Autodesk Inventor part; units mm, degrees
ref_plane "YZ Plane" through (0, 0, 0) normal (1, 0, 0) x (0, 1, 0)
ref_plane "XZ Plane" through (0, 0, 0) normal (0, 1, 0) x (-1, 0, 0)
ref_plane "XY Plane" through (0, 0, 0) normal (0, 0, 1) x (1, 0, 0)
sketch "Sketch1" plane through (0, 0, 0) normal (0, 1, 0) x (-1, 0, 0)
  line L0 (0, 0) -> (0, -34.15) construction
  arc A0 (6.6649, -3.975) -> (-7.575, -7.575) centre (0, -7.575) ccw construction
  arc A1 (-7.575, -26.575) -> (6.6649, -30.175) centre (0, -26.575) ccw construction
  line L1 (4.075, -7.575) -> (4.075, -26.575) construction
  arc A2 (-4.075, -26.575) -> (4.075, -26.575) centre (0, -26.575) ccw construction
  line L2 (-4.075, -26.575) -> (-4.075, -7.575) construction
  arc A3 (4.075, -7.575) -> (-4.075, -7.575) centre (0, -7.575) ccw construction
  line L3 (9.1649, -3.975) -> (9.1649, -30.175) construction
  line L4 (9.1649, -3.975) -> (6.6649, -3.975) construction
  line L5 (9.1649, -30.175) -> (6.6649, -30.175) construction
  line L6 (-10.575, -14.075) -> (-10.575, -20.075) construction
  line L7 (0, -17.075) -> (-19.3792, -17.075) construction
  line L8 (-4.075, -20.075) -> (-4.075, -24.075) construction
  line L9 (-10.575, -20.075) -> (-7.575, -21.8932) construction
  line L10 (-10.575, -14.075) -> (-7.575, -12.2568) construction
  line L11 (-7.575, -7.575) -> (-7.575, -12.2568) construction
  line L12 (-7.575, -21.8932) -> (-7.575, -26.575) construction
  line L13 (-10.575, -17.075) -> (-16.875, -17.075) construction
  line L14 (-10.575, -14.075) -> (-14.875, -14.075) construction
  line L15 (-16.875, -16.075) -> (-16.875, -18.075) construction
  line L16 (-14.875, -20.075) -> (-10.575, -20.075) construction
  arc A4 (-14.875, -14.075) -> (-16.875, -16.075) centre (-14.875, -16.075) ccw construction
  arc A5 (-16.875, -18.075) -> (-14.875, -20.075) centre (-14.875, -18.075) ccw construction
  line L17 (-6.7059, -17.075) -> (-6.7059, -23.075) construction
  line L18 (-6.7059, -17.075) -> (-6.7059, -11.075) construction
  line L19 (-7.575, -11.075) -> (-14.875, -11.075) construction
  line L20 (-16.875, -13.075) -> (-16.875, -21.075) construction
  line L21 (-14.875, -23.075) -> (-7.575, -23.075) construction
  arc A6 (-14.875, -11.075) -> (-16.875, -13.075) centre (-14.875, -13.075) ccw construction
  arc A7 (-16.875, -21.075) -> (-14.875, -23.075) centre (-14.875, -21.075) ccw construction
  line L22 (19.3047, -16.075) -> (19.3047, -18.075) construction
  line L23 (17.3047, -14.075) -> (13.3047, -14.075) construction
  line L24 (17.3047, -20.075) -> (13.3047, -20.075) construction
  line L25 (9.1649, -16.075) -> (9.1649, -22.575) construction
  line L26 (9.1649, -17.075) -> (9.1649, -11.575) construction
  line L27 (9.1649, -11.575) -> (13.3047, -14.075) construction
  line L28 (9.1649, -22.575) -> (13.3047, -20.075) construction
  arc A8 (19.3047, -16.075) -> (17.3047, -14.075) centre (17.3047, -16.075) ccw construction
  arc A9 (17.3047, -20.075) -> (19.3047, -18.075) centre (17.3047, -18.075) ccw construction
  line L29 (9.1649, -30.175) -> (9.1649, -26.175) construction
  line L30 (9.1649, -3.975) -> (9.1649, -7.975) construction
  line L31 (9.1649, -24.9114) -> (13.8618, -22.075) construction
  line L32 (13.8618, -22.075) -> (17.3047, -22.075) construction
  arc A10 (17.3047, -22.075) -> (21.3047, -18.075) centre (17.3047, -18.075) ccw construction
  line L33 (21.3047, -18.075) -> (21.3047, -16.075) construction
  arc A11 (21.3047, -16.075) -> (17.3047, -12.075) centre (17.3047, -16.075) ccw construction
  line L34 (17.3047, -12.075) -> (13.8618, -12.075) construction
  line L35 (13.8618, -12.075) -> (9.1649, -9.2386) construction
  point P0 (7.575, -17.075)
  point P1 (-4.075, -10.075)
  point P2 (19.3047, -14.075)
  point P3 (19.3047, -20.075)
  dimension "d0" = 34.15
  dimension "d1" = 15.15
  dimension "d5" = 6
  dimension "d7" = 4
  dimension "d8" = 2.5
  dimension "d9" = 3.5
  dimension "d10" = 8.15
  dimension "d12" = 2
  dimension "d14" = 6
  dimension "d15" = 6
  dimension "d16" = 2
  dimension "d18" = 6
  dimension "d19" = 6
  dimension "d20" = 5.5
  dimension "d21" = 5.5
  dimension "d23" = 4
  dimension "d24" = 4
  dimension "d25" = 2
sketch "Sketch3" plane through (0, 0, 0) normal (0, 1, 0) x (-1, 0, 0)
  arc A0 (6.6649, -3.975) -> (-7.575, -7.575) centre (0, -7.575) ccw construction
  arc A1 (-7.575, -26.575) -> (6.6649, -30.175) centre (0, -26.575) ccw construction
  arc A2 (-4.075, -26.575) -> (4.075, -26.575) centre (0, -26.575) ccw
  line L0 (4.075, -7.575) -> (4.075, -26.575)
  arc A3 (4.075, -7.575) -> (-4.075, -7.575) centre (0, -7.575) ccw
  line L1 (-4.075, -26.575) -> (-4.075, -7.575)
  line L2 (9.1649, -3.975) -> (9.1649, -30.175) construction
  line L3 (-10.575, -14.075) -> (-10.575, -20.075) construction
  line L4 (-16.875, -16.075) -> (-16.875, -18.075) construction
  arc A4 (8.836, -1.765) -> (-4.3309, 2.0725) centre (0, -7.575) ccw
  arc A5 (-4.3309, -36.2225) -> (8.836, -32.385) centre (0, -26.575) ccw
  line L5 (9.1649, -2.8638) -> (9.1649, -31.2862)
  arc A6 (9.1649, -2.8638) -> (8.836, -1.765) centre (7.1649, -2.8638) ccw
  arc A7 (8.836, -32.385) -> (9.1649, -31.2862) centre (7.1649, -31.2862) ccw
  line L6 (-12.075, -10.8843) -> (-12.075, -24.6972)
  ellipse E0 centre (0, -17.075) end of major axis (0, -37.15) minor radius 14.4147 (-4.3309, 2.0725) -> (-4.3309, -36.2225) ccw
  point P0 (0, 0)
  point P1 (9.1649, -2.2991)
  point P2 (9.1649, -31.8509)
  dimension "d26" = 3
  dimension "d27" = 3
  dimension "d28" = 2
  dimension "d29" = 6.5
  dimension "d30" = 8
extrude "Extrusion1" add sketch "Sketch3" along normal blind 1
ref_plane "Work Plane1" through (0, 1, 3) normal (1, 0, 0) x (0, 0, -1)
sketch "Sketch7" plane through (0, 1, 3) normal (1, 0, 0) x (0, 0, -1)
  line L0 (40.15, 0) -> (40.15, -1)
  line L1 (40.15, -1) -> (33.65, -1)
  line L2 (33.65, -1) -> (33.65, 0)
  line L3 (33.65, 0) -> (40.15, 0)
  line L4 (0, -1) -> (0, 0)
  line L5 (0, 0) -> (6.5, 0)
  line L6 (6.5, 0) -> (6.5, -1)
  line L7 (6.5, -1) -> (0, -1)
  line L8 (40.15, -1) -> (35.385, -1) construction
  line L9 (40.15, -1) -> (40.15, -0.5) construction
  line L10 (40.15, -1) -> (40.15, 0) construction
  line L11 (4.765, 0) -> (0, 0) construction
  line L12 (40.15, -0.5) -> (0, 0)
  line L13 (0, 0) -> (40.15, 0)
  line L14 (40.15, 0) -> (40.15, -0.5)
  point P0 (3, -1)
  point P1 (39.2225, -1)
  point P2 (0.9275, 0)
extrude "Extrusion2" cut sketch "Sketch7" along normal blind 20 and the other way blind 20 contours L0 L12 L2 L3 | L2 L12 L6 L13 | L6 L12 L5
properties part number "SPD_MTB_cleat_new_1mm_05mm"
Here's how the part is built. I have some questions about the finished solid (model axes, mm). A direction names the side the tool comes from. Coordinates: 2 decimals unless noted, no trailing zeros. Order: outer loops, then holes, each group sorted by start corner. A loop starts at its lowest first (then second) coordinate and runs counter-clockwise, first axis right, second up.
Item 1: I need wall thicknesses on probe 1 along Z at (x, y) = (0, 0.45); probe 2 along X at (y, z) = (0.85, -5.5); probe 3 along X at (y, z) = (0.25, -19) (3 decimals). Which ranges of each line are inside material? Lowest first, please.
Response values:
probe 1: z = -37.15 to -30.65, -3.5 to 3
probe 2: x = -9.16 to -3.51, 3.51 to 11.78
probe 3: x = -9.165 to -4.075, 4.075 to 14.348
Item 2: Which directions (+Z, -Z, +X, -X, +Y, -Y) give clear straight access to the entire face, cutting with the end or side of a thin tool? Please do faces 5 (the face through (-9.165, 0.4, -16.9)), 6 (the face through (-4.075, 0.3, -16.9)).
Response values:
face 5: +Z, -Z, -X, +Y, -Y
face 6: +Y, -Y
Item 3: Thinking about a two-plate mould opening in X: for faces 1 (the face through (-9.079, 0.464, -2.283)), 2 (the face through (-2.859, 0.493, 2.606)), 3 (the face through (4.075, 0.3, -17.2)), 4 (the face through (5, 0, -17)), which applies, pulls with the +X half, pulls with the -X half, needs draft (parallel to the pull), parting line crosses it, or undercut?
Response values:
face 1: pulls with the -X half
face 2: parting line crosses it
face 3: undercut
face 4: needs draft
Item 4: If we section it at A-A, the plane x = -3: List the corners of the cut face in (y, z) for me.
Response values:
outline: (0, -36.72) - (0.51, -36.72) - (0.6, -29.33) - (0, -29.33) - close; (0, -4.82) - (0.9, -4.82) - (0.99, 2.57) - (0, 2.57) - close
